Check sheet for the drawn part. Datum: minimum x, y, z corner. Units: mm. Round coordinates to 2 decimals unless told otherwise and drop trailing zeros. Write each loop counter-clockwise with the first axis right and the second up, starting at its lowest first coordinate (ties: lowest second). Pieces come first, ordered by that corner, then holes.
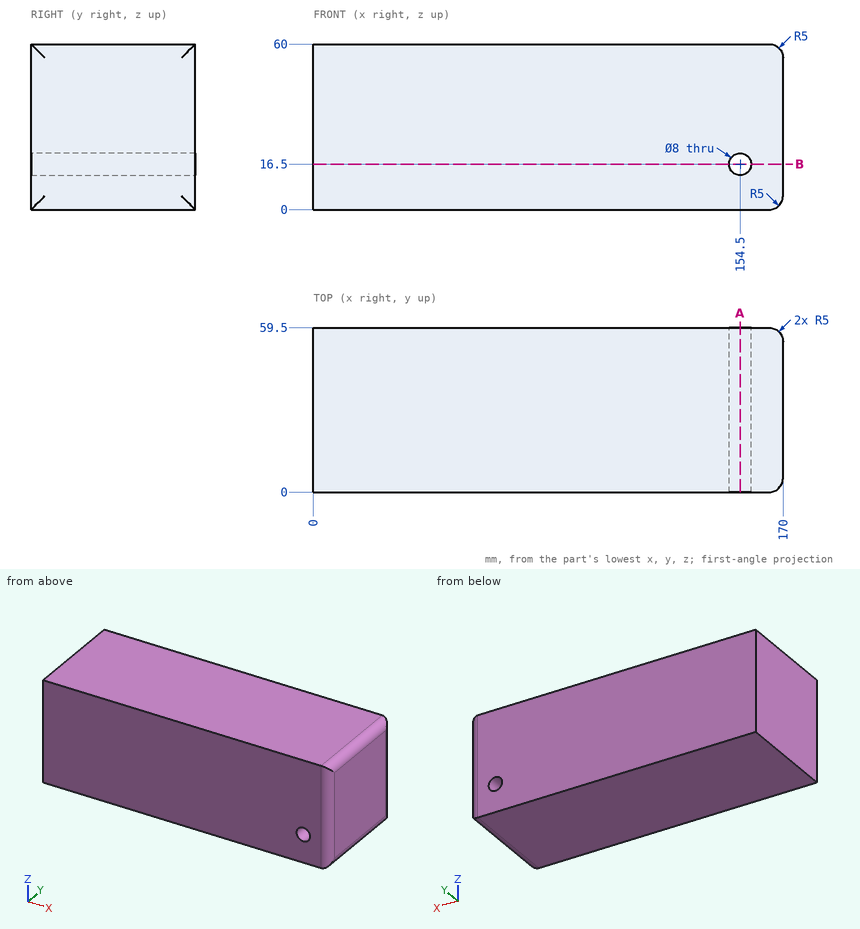
Q1. Material ranges on line 1 along X through (y, z) = (47.5, 17); line 2 along Z through (x, y) = (154, 26); line 3 along X through (y, z) = (22.5, 17.5), recorded low to high.
Recorded:
line 1: x = 0 to 150.53, 158.47 to 170
line 2: z = 0 to 12.53, 20.47 to 60
line 3: x = 0 to 150.63, 158.37 to 170
Q2. Sectioned sample at A-A (x = 154.5). Enter the section's corners in (y, z).
Recorded:
outline: (0, 0) - (59.5, 0) - (59.5, 12.5) - (0, 12.5) - close; (0, 20.5) - (59.5, 20.5) - (59.5, 60) - (0, 60) - close
Q3. Sectioned sample at B-B (z = 16.5). Enter the section's corners in (x, y).
Recorded:
outline: (0, 0) - (150.5, 0) - (150.5, 59.5) - (0, 59.5) - close; (158.5, 0) - (165, 0) arc R5 ccw to (170, 5) - (170, 54.5) arc R5 ccw to (165, 59.5) - (158.5, 59.5) - close
